```python
from build123d import *

# Parameters (mm, degrees)
SKETCH2_R                = 22.849514629
BOSS_EXTRUDE4_DEPTH      = 3
BOSS_EXTRUDE5_DEPTH      = 2
BOSS_EXTRUDE6_DEPTH      = 3
BOSS_EXTRUDE6_DEPTH_BACK = 0.5


with BuildPart() as part:
    # Sketch2 → Boss-Extrude4 (new body)
    with BuildSketch(Plane(origin=(0, 0, 0), x_dir=(1, 0, 0), z_dir=(0, 1, 0))):
        with BuildLine():
            Line((-5.466491508, -28.085827415), (-5.466491508, -31.529628456))
            ThreePointArc((-5.466491508, -31.529628456), (-27.820132871, -15.812659708), (-29.887127171, 11.435017686))
            Line((-29.887127171, 11.435017686), (-26.843313916, 9.677671284))
            Line((-26.843313916, 9.677671284), (-21.589794274, 18.777034223))
            Line((-21.589794274, 18.777034223), (-24.572213461, 20.498934743))
            ThreePointArc((-24.572213461, 20.498934743), (0.215901427, 31.999271657), (24.846579394, 20.165502533))
            Line((24.846579394, 20.165502533), (21.802766139, 18.408156131))
            Line((21.802766139, 18.408156131), (27.056285781, 9.308793192))
            Line((27.056285781, 9.308793192), (30.038704969, 11.030693713))
            ThreePointArc((30.038704969, 11.030693713), (27.604231444, -16.186611949), (5.040547776, -31.600520219))
            Line((5.040547776, -31.600520219), (5.040547776, -28.085827415))
            Line((5.040547776, -28.085827415), (-5.466491508, -28.085827415))
        make_face()
        Circle(SKETCH2_R, mode=Mode.SUBTRACT)
    extrude(amount=BOSS_EXTRUDE4_DEPTH)

    # Sketch2_12 → Boss-Extrude5 (add)
    with BuildSketch(Plane(origin=(0, 0, 0), x_dir=(1, 0, 0), z_dir=(0, 1, 0))):
        with BuildLine():
            Line((-5.466491508, -31.529628456), (-5.466491508, -28.085827415))
            Line((-5.466491508, -28.085827415), (5.040547776, -28.085827415))
            Line((5.040547776, -28.085827415), (5.040547776, -31.600520219))
            ThreePointArc((5.040547776, -31.600520219), (27.604231444, -16.186611949), (30.038704969, 11.030693713))
            Line((30.038704969, 11.030693713), (27.056285781, 9.308793192))
            Line((27.056285781, 9.308793192), (21.802766139, 18.408156131))
            Line((21.802766139, 18.408156131), (24.846579394, 20.165502533))
            ThreePointArc((24.846579394, 20.165502533), (0.215901427, 31.999271657), (-24.572213461, 20.498934743))
            Line((-24.572213461, 20.498934743), (-21.589794274, 18.777034223))
            Line((-21.589794274, 18.777034223), (-26.843313916, 9.677671284))
            Line((-26.843313916, 9.677671284), (-29.887127171, 11.435017686))
            ThreePointArc((-29.887127171, 11.435017686), (-27.820132871, -15.812659708), (-5.466491508, -31.529628456))
        make_face()
        with BuildLine():
            ThreePointArc((2.502594182, -22.712052772), (0, -22.849514629), (-2.502594182, -22.712052772))
            ThreePointArc((-2.502594182, -22.712052772), (-19.788260133, -11.424757314), (-20.920511764, 9.188716249))
            ThreePointArc((-20.920511764, 9.188716249), (-19.788260133, 11.424757314), (-18.417917582, 13.523336524))
            ThreePointArc((-18.417917582, 13.523336524), (0, 22.849514629), (18.417917582, 13.523336524))
            ThreePointArc((18.417917582, 13.523336524), (19.788260133, 11.424757314), (20.920511764, 9.188716249))
            ThreePointArc((20.920511764, 9.188716249), (22.362064511, 4.69450632), (22.849514629, 0))
            ThreePointArc((22.849514629, 0), (17.018862787, -15.246593987), (2.502594182, -22.712052772))
        make_face(mode=Mode.SUBTRACT)
    extrude(amount=-BOSS_EXTRUDE5_DEPTH)

    # Sketch2_13 → Boss-Extrude6 (add, two sides)
    with BuildSketch(Plane(origin=(0, 0, 0), x_dir=(1, 0, 0), z_dir=(0, 1, 0))) as boss_extrude6_sk:
        with BuildLine():
            Line((2.502594182, -22.112052772), (-2.502594182, -22.112052772))
            Line((-2.502594182, -22.112052772), (-2.502594182, -22.712052772))
            ThreePointArc((-2.502594182, -22.712052772), (0, -22.849514629), (2.502594182, -22.712052772))
            Line((2.502594182, -22.712052772), (2.502594182, -22.112052772))
        make_face()
        with BuildLine():
            ThreePointArc((-18.417917582, 13.523336524), (-19.788260133, 11.424757314), (-20.920511764, 9.188716249))
            Line((-20.920511764, 9.188716249), (-20.400896522, 8.888716249))
            Line((-20.400896522, 8.888716249), (-17.89830234, 13.223336524))
            Line((-17.89830234, 13.223336524), (-18.417917582, 13.523336524))
        make_face()
        with BuildLine():
            Line((20.400896522, 8.888716249), (20.920511764, 9.188716249))
            ThreePointArc((20.920511764, 9.188716249), (19.788260133, 11.424757314), (18.417917582, 13.523336524))
            Line((18.417917582, 13.523336524), (17.89830234, 13.223336524))
            Line((17.89830234, 13.223336524), (20.400896522, 8.888716249))
        make_face()
    extrude(amount=BOSS_EXTRUDE6_DEPTH)
    extrude(boss_extrude6_sk.sketch, amount=-BOSS_EXTRUDE6_DEPTH_BACK)


solid = part.part
```
Design review of the part built by this model. Coordinates are the model's own, in mm. A direction names the side the tool comes from. Round coordinates to 2 decimals unless told otherwise and drop trailing zeros. Write each loop counter-clockwise with the first axis right and the second up, starting at its lowest first coordinate (ties: lowest second). Pieces come first, ordered by that corner, then holes.
Item 1: We need section C-C on x = 8.5. Write out the cut boundary in (y, z).
Item 2: We need section B-B on y = 1.2. Write out the cut boundary in (x, z).
Item 3: Clearance check with flat-ended pins moving along their axes: pin 1 Ø12 at (x, z) = (12.5, -9) entering from -Y; pin 2 Ø3 at (x, y) = (-12.5, 2) entering from -Z; pin 3 Ø2 at (x, y) = (-24.5, 0.5) entering from +Z; pin 4 Ø3 at (y, z) = (-0.5, 7) entering from -X. State where each tip first meets the part, or that it passes through.
Item 4: The part is to be moulded in two halves that separate along Z. For faces 1 (the flat face through (-19.4, -0.5, -11.2)), 2 (the cylindrical face through (27.4, 0.54, 16.53)), 3 (the cylindrical face through (0.611, 0.535, -31.994)), say which applies: +Z half, -Z half, draft (parallel to the pull), parting line (faces both ways), or undercut.
Item 5: For faces 4 (the flat face through (28.6, 0.5, -10.2)), 5 (the flat face through (-23.1, 0.54, -19.65)), 6 (the flat face through (23.303, 0.535, -19.275)), 7 (the flat face through (-24.18, 0.54, -14.29)), 8 (the flat face through (19.4, -0.5, -11.2)), list the 3-axis set-ups (+Z, -Z, +X, -X, +Y, -Y) from which the entire face can be reached by the end or side of a thin tool; tool diameter is ignored.
Item 6: For probe 1 along Z at (x, y) = (-3.5, 0.4); probe 2 along X at (y, z) = (0, 0); probe 3 along X at (y, z) = (-1.8, -12), list the stretches that pass through material, from the lowest coordinate up.
Item 7: We need section A-A on z = 2. Write out the cut boundary in (x, y).
Item 8: We need section D-D on x = 24. Write out the cut boundary in (y, z).
Returned:
1. outline: (-2, -30.85) - (3, -30.85) - (3, -21.21) - (-2, -21.21) - close; (-2, 21.21) - (3, 21.21) - (3, 30.85) - (-2, 30.85) - close
2. outline: (-29.89, -11.44) - (-26.84, -9.68) - (-21.59, -18.78) - (-24.57, -20.5) arc R32 ccw to (24.85, -20.17) - (21.8, -18.41) - (27.06, -9.31) - (30.04, -11.03) arc R32 ccw to (5.04, 31.6) - (5.04, 28.09) - (-5.47, 28.09) - (-5.47, 31.53) arc R32 ccw to start; hole (-20.92, -9.19) - (-20.4, -8.89) - (-17.9, -13.22) - (-18.42, -13.52) arc R22.85 ccw to (18.42, -13.52) - (17.9, -13.22) - (20.4, -8.89) - (20.92, -9.19) arc R22.85 ccw to (2.5, 22.71) - (2.5, 22.11) - (-2.5, 22.11) - (-2.5, 22.71) arc R22.85 ccw to start
3. pin 1: passes through
3. pin 2: stops at z = -30.05
3. pin 3: stops at z = 21.72
3. pin 4: stops at x = -31.52
4. face 1: undercut
4. face 2: parting line
4. face 3: -Z half
5. face 4: -Z, +Y, -Y
5. face 5: -X, +Y, -Y
5. face 6: +X, +Y, -Y
5. face 7: +Y, -Y
5. face 8: -Y
6. probe 1: z = -31.81 to -22.58, 22.58 to 28.09
6. probe 2: x = -32 to -22.85, 22.85 to 32
6. probe 3: x = -25.5 to -19.44, 19.44 to 25.5
7. outline: (-31.94, -2) - (-22.76, -2) - (-22.76, 3) - (-31.94, 3) - close; (22.76, -2) - (31.94, -2) - (31.94, 3) - (22.76, 3) - close
8. outline: (-2, -21.17) - (3, -21.17) - (3, -19.68) - (-2, -19.68) - close; (-2, -14.6) - (3, -14.6) - (3, 21.17) - (-2, 21.17) - close
